For this review, take the finished solid that the model builds, in its own axes (mm). A direction names the side the tool comes from. Coordinates: 2 decimals unless noted, no trailing zeros. Write each loop counter-clockwise with the first axis right and the second up, starting at its lowest first coordinate (ties: lowest second). Pieces come first, ordered by that corner, then holes. Notation, with made-up numbers: M 17,-17 L 25,-17 A20 ccw 25,11 Z; hole C -30,27.5 d5. An arc over 180 degrees is marked long. One line per question, with ' | ' between items.
from build123d import *

# Parameters (mm, degrees)
SKETCH1_W           = 45
SKETCH1_H           = 250
BOSS_EXTRUDE1_DEPTH = 12
SKETCH2_R           = 2.5
SKETCH2_R_2         = 5
SKETCH2_W           = 5
SKETCH2_H           = 105
SKETCH2_W_2         = 45
SKETCH2_H_2         = 15
CUT_EXTRUDE1_DEPTH  = 12
SKETCH3_R           = 1.75
CUT_EXTRUDE2_DEPTH  = 35
SKETCH4_W           = 25
SKETCH4_H           = 12
BOSS_EXTRUDE2_DEPTH = 12
SKETCH5_W           = 45
SKETCH5_H           = 23
CUT_EXTRUDE3_DEPTH  = 20
SKETCH6_W           = 70
SKETCH6_H           = 7
BOSS_EXTRUDE3_DEPTH = 12
SKETCH7_R           = 1.5
CUT_EXTRUDE4_DEPTH  = 12
CUT_EXTRUDE5_DEPTH  = 20
FILLET1_R           = 18
SKETCH9_R           = 11
CUT_EXTRUDE6_DEPTH  = 7


with BuildPart() as part:
    # Sketch1 → Boss-Extrude1 (new body)
    with BuildSketch(Plane(origin=(0, 0, 0), x_dir=(1, 0, 0), z_dir=(0, 1, 0))):
        Rectangle(SKETCH1_W, SKETCH1_H)
    extrude(amount=BOSS_EXTRUDE1_DEPTH)

    # Sketch2 → Cut-Extrude1 (cut)
    with BuildSketch(Plane(origin=(0, 12, 0), x_dir=(1, 0, 0), z_dir=(0, 1, 0))):
        with Locations(Location((0, 12, 0), (0, 0, 270))):
            Circle(SKETCH2_R)
        with Locations(Location((0, 30.25, 0), (0, 0, 270))):
            Circle(SKETCH2_R_2)
        with Locations(Location((0, 48.5, 0), (0, 0, 270))):
            Circle(SKETCH2_R)
        with Locations(Location((0, -67.5, 0), (0, 0, 270))):
            Circle(SKETCH2_R_2)
        with Locations((20, 60.5)):
            Rectangle(SKETCH2_W, SKETCH2_H)
        with Locations((-20, 60.5)):
            Rectangle(SKETCH2_W, SKETCH2_H)
        with Locations((0, -117.5)):
            Rectangle(SKETCH2_W_2, SKETCH2_H_2)
    extrude(amount=-CUT_EXTRUDE1_DEPTH, mode=Mode.SUBTRACT)

    # Sketch3 → Cut-Extrude2 (cut)
    with BuildSketch(Plane(origin=(17.5, 0, 0), x_dir=(0, 0, -1), z_dir=(1, 0, 0))):
        with Locations((33, 5)):
            Circle(SKETCH3_R)
        with Locations((65.5, 5)):
            Circle(SKETCH3_R)
        with Locations((105.5, 5)):
            Circle(SKETCH3_R)
    extrude(amount=-CUT_EXTRUDE2_DEPTH, mode=Mode.SUBTRACT)

    # Sketch4 → Boss-Extrude2 (add)
    with BuildSketch(Plane(origin=(0, 12, 0), x_dir=(1, 0, 0), z_dir=(0, 1, 0))):
        with Locations((35, 119)):
            Rectangle(SKETCH4_W, SKETCH4_H)
    extrude(amount=-BOSS_EXTRUDE2_DEPTH)

    # Sketch5 → Cut-Extrude3 (cut)
    with BuildSketch(Plane(origin=(0, 12, 0), x_dir=(1, 0, 0), z_dir=(0, 1, 0))):
        with Locations((0, -98.5)):
            Rectangle(SKETCH5_W, SKETCH5_H)
    extrude(amount=-CUT_EXTRUDE3_DEPTH, mode=Mode.SUBTRACT)

    # Sketch6 → Boss-Extrude3 (add)
    with BuildSketch(Plane(origin=(0, 12, 0), x_dir=(1, 0, 0), z_dir=(0, 1, 0))):
        with Locations((12.5, 128.5)):
            Rectangle(SKETCH6_W, SKETCH6_H)
    extrude(amount=-BOSS_EXTRUDE3_DEPTH)

    # Sketch7 → Cut-Extrude4 (cut)
    with BuildSketch(Plane(origin=(0, 12, 0), x_dir=(1, 0, 0), z_dir=(0, 1, 0))):
        with Locations(Location((38, 122.5, 0), (0, 0, 270))):
            Circle(SKETCH7_R)
        with Locations(Location((44, 122.5, 0), (0, 0, 270))):
            Circle(SKETCH7_R)
    extrude(amount=-CUT_EXTRUDE4_DEPTH, mode=Mode.SUBTRACT)

    # Sketch8 → Cut-Extrude5 (cut)
    with BuildSketch(Plane(origin=(0, 12, 0), x_dir=(1, 0, 0), z_dir=(0, 1, 0))):
        Polygon((-22.5, -2), (-22.5, -87), (-17.5, -87), align=None)
        Polygon((17.5, -87), (22.5, -2), (22.5, -87), align=None)
    extrude(amount=-CUT_EXTRUDE5_DEPTH, mode=Mode.SUBTRACT)

    # Fillet1
    fillet1_edges = [part.edges().sort_by_distance(p)[0] for p in [
        (17.5, 6, 87),
        (-17.5, 6, 87),
    ]]
    fillet(fillet1_edges, radius=FILLET1_R)

    # Sketch9 → Cut-Extrude6 (cut)
    with BuildSketch(Plane.XZ):
        with Locations(Location((0, 67.5, 0), (0, 0, 270))):
            Circle(SKETCH9_R)
    extrude(amount=-CUT_EXTRUDE6_DEPTH, mode=Mode.SUBTRACT)


solid = part.part
1. For line 1 along Y through (x, z) = (-2, -105.5); line 2 along X through (y, z) = (7.25, -122.5); line 3 along X through (y, z) = (7.75, -18), list the stretches that pass through material, from the lowest coordinate up.
Computed values:
line 1: y = 0 to 3.25, 6.75 to 12 | line 2: x = -22.5 to 36.5, 39.5 to 42.5, 45.5 to 47.5 | line 3: x = -17.5 to 17.5
2. Take a section at B-B on x = 7. State the section outline as (y, z) points, plus the area to 3 significant figures.
Computed values:
outline: M 0,-132 L 12,-132 L 12,85.8 L 0,85.8 L 0,75.99 L 7,75.99 L 7,59.01 L 0,59.01 Z; hole C 5,-105.5 d3.5; hole C 5,-65.5 d3.5; hole C 5,-33 d3.5 | area: 2,470 mm2
3. Take a section at A-A on z = -12. State the section outline as (x, y) points.
Computed values:
outline: M -17.5,0 L -2.5,0 L -2.5,12 L -17.5,12 Z; M 2.5,0 L 17.5,0 L 17.5,12 L 2.5,12 Z
4. Clearance check with flat-ended pins moving along their axes: P1, Ø4, axis at y = 2, z = -20.5, coming from the -X side; P2, Ø4, axis at x = -19, y = 5.5, coming from the +Z side; P3, Ø6.5, axis at x = 0, z = -48.5, coming from the +Y side; P4, Ø13, axis at x = 0, z = 67.5, coming from the -Y side. State where each tip first meets the part, or that it passes through.
Computed values:
P1: stops at x = -17.5 | P2: stops at z = 76.26 | P3: stops at y = 12 | P4: stops at y = 7
5. Take a section at D-D on x = -9. State the section outline as (y, z) points, plus the area to 3 significant figures.
Computed values:
outline: M 0,-132 L 12,-132 L 12,84.88 L 0,84.88 L 0,73.82 L 7,73.82 L 7,61.18 L 0,61.18 Z; hole C 5,-105.5 d3.5; hole C 5,-65.5 d3.5; hole C 5,-33 d3.5 | area: 2,490 mm2
6. Draft analysis for pull direction X (two halves, no side actions). For faces 5 (the flat face through (4, 0, -24)), 6 (the cylindrical face through (-1.915, 9.535, 72.119)), 7 (the flat face through (47.5, 6, -122)), state which applies: pulls with the +X half, pulls with the -X half, needs draft (parallel to the pull), parting line crosses it, or undercut.
Computed values:
face 5: needs draft | face 6: undercut | face 7: pulls with the +X half
7. Machinability: for faces 1 (the flat face through (17.5, 6, -60)), 2 (the flat face through (-20, 6, -113)), 3 (the flat face through (-5, 7, 65)), 4 (the flat face through (22.5, 6, -3)), which of the approach directions +Z, -Z, +X, -X, +Y, -Y give a long, thin tool a straight path to every point of the face, cutting with its end or side? Answer none if there is none.
Computed values:
face 1: +X, +Y, -Y | face 2: -X, +Y, -Y | face 3: -Y | face 4: +Z, +X, +Y, -Y
8. Take a section at C-C on z = -95. State the section outline as (x, y) points, plus the area to 3 significant figures.
Computed values:
outline: M -17.5,0 L 17.5,0 L 17.5,12 L -17.5,12 Z | area: 420 mm2
